Source: CAD feature listing. Evaluate the final solid. Frame: model axes, mm. Round coordinates to 2 decimals unless told otherwise and drop trailing zeros. Order: outer loops, then holes, each group sorted by start corner. A loop starts at its lowest first (then second) coordinate and runs counter-clockwise, first axis right, second up. Notation, with made-up numbers: M 18.25,7 L 68.25,7 A13 cw 68.25,26 Z; hole C 6,76.25 d1. An arc over 180 degrees is marked long. Use one line per item in the form item = value. Start each with the question number.
Q1. Section B-B (x = -12.7). Return the cut outline in (y, z), plus the area to 3 significant figures.
Q2. Material intervals for probe 1 along Z at (x, y) = (-12.7, 1.5); probe 2 along X at (y, z) = (2.5, -57.15) (3 decimals); probe 3 along X at (y, z) = (2.5, 44.45), sorted ascending.
Q3. Section A-A (z = 38.1). Return the cut outline in (x, y), plus the area to 3 significant figures.
from build123d import *

# Parameters (mm, degrees)
SKETCH1_W                  = 88.9
SKETCH1_H                  = 127
BOSS_EXTRUDE1_DEPTH        = 6.35
F_1_4_0_2500_DOWEL_HOLE1_D = 6.35
F_8_32_TAPPED_HOLE1_D      = 3.4544
F_1_4_0_2500_DOWEL_HOLE2_D = 6.35
F_8_32_TAPPED_HOLE2_D      = 3.4544


with BuildPart() as part:
    # Sketch1 → Boss-Extrude1 (new body)
    with BuildSketch(Plane(origin=(0, 0, 0), x_dir=(1, 0, 0), z_dir=(0, 1, 0))):
        Rectangle(SKETCH1_W, SKETCH1_H)
    extrude(amount=BOSS_EXTRUDE1_DEPTH)

    # 1/4 (0.2500) Dowel Hole1 (through all)
    with Locations(Plane(origin=(0, 6.35, 0), x_dir=(1, 0, 0), z_dir=(0, 1, 0))):
        with Locations((-22.225, -44.45), (-22.225, 44.45)):
            Hole(F_1_4_0_2500_DOWEL_HOLE1_D / 2)

    # #8-32 Tapped Hole1 (through all)
    with Locations(Plane(origin=(0, 6.35, 0), x_dir=(1, 0, 0), z_dir=(0, 1, 0))):
        with Locations((-9.525, -38.1), (-9.525, 38.1)):
            Hole(F_8_32_TAPPED_HOLE1_D / 2)

    # 1/4 (0.2500) Dowel Hole2 (through all)
    with Locations(Plane(origin=(0, 6.35, 0), x_dir=(1, 0, 0), z_dir=(0, 1, 0))):
        with Locations((-19.05, 57.15), (-19.05, -57.15)):
            Hole(F_1_4_0_2500_DOWEL_HOLE2_D / 2)

    # #8-32 Tapped Hole2 (through all)
    with Locations(Plane(origin=(0, 6.35, 0), x_dir=(1, 0, 0), z_dir=(0, 1, 0))):
        with Locations((-12.7, 50.8), (-12.7, -50.8)):
            Hole(F_8_32_TAPPED_HOLE2_D / 2)


solid = part.part
Results list:
q1.outline = M 0,-63.5 L 6.35,-63.5 L 6.35,-52.53 L 0,-52.53 Z; M 0,-49.07 L 6.35,-49.07 L 6.35,49.07 L 0,49.07 Z; M 0,52.53 L 6.35,52.53 L 6.35,63.5 L 0,63.5 Z
q1.area = 763 mm2
q2.probe_1 = -63.5 to -52.53, -49.07 to 49.07, 52.53 to 63.5
q2.probe_2 = -44.45 to -22.225, -15.875 to 44.45
q2.probe_3 = -44.45 to -25.4, -19.05 to 44.45
q3.outline = M -44.45,0 L -11.25,0 L -11.25,6.35 L -44.45,6.35 Z; M -7.8,0 L 44.45,0 L 44.45,6.35 L -7.8,6.35 Z
q3.area = 543 mm2
